Source: CAD feature listing. Evaluate the final solid. Frame: model axes, mm. Face numbers are marked on the shaded views. A direction names the side the tool comes from. Round coordinates to 2 decimals unless told otherwise and drop trailing zeros. Write each loop counter-clockwise with the first axis right and the second up, starting at its lowest first coordinate (ties: lowest second). Pieces come first, ordered by that corner, then holes. Notation, with made-up numbers: M -2.75,-22.5 L 19.25,-22.5 A34 ccw 19.25,12.5 Z; hole C 13,56 d4. An arc over 180 degrees is marked long. Answer in a Markdown table with one row per item.
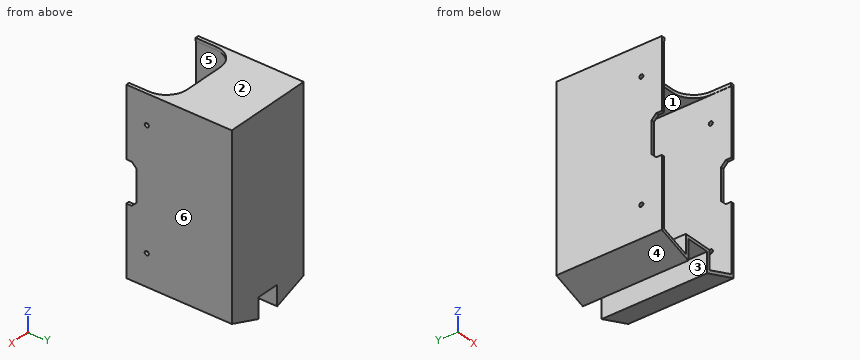
from build123d import *

# Parameters (mm, degrees)
BOSS_EXTRUDE1_DEPTH = 50
BOSS_EXTRUDE2_DEPTH = 1.52
CUT_EXTRUDE2_DEPTH  = 1.52
SKETCH4_R           = 1
CUT_EXTRUDE8_DEPTH  = 178.52
CUT_EXTRUDE9_DEPTH  = 178.52


with BuildPart() as part:
    # Sketch1 → Boss-Extrude1 (new body)
    with BuildSketch(Plane(origin=(0, 0, 0), x_dir=(1, 0, 0), z_dir=(0, 1, 0))):
        Polygon((-22.935245878, -45.076760645), (20.864754122, -45.076760645), (20.864754122, 42.660744493), (4.698193973, 48.553690828), (4.698193973, 38.723239355), (-6.768685729, 38.723239355), (-6.768685729, 48.553690828), (-22.935245878, 42.660744493), align=None)
        Polygon((-21.435245878, -43.576760645), (19.364754122, -43.576760645), (19.364754122, 41.610970221), (6.198193973, 46.410372917), (6.198193973, 37.223239355), (-8.268685729, 37.223239355), (-8.268685729, 46.410372917), (-21.435245878, 41.610970221), align=None, mode=Mode.SUBTRACT)
    extrude(amount=BOSS_EXTRUDE1_DEPTH)

    # Sketch2 → Boss-Extrude2 (add)
    with BuildSketch(Plane(origin=(0, 50, 0), x_dir=(1, 0, 0), z_dir=(0, 1, 0))):
        Polygon((-22.935245878, 42.660744493), (-22.935245878, -45.076760645), (20.864754122, -45.076760645), (20.864754122, 42.660744493), (4.698193973, 48.553690828), (4.698193973, 38.723239355), (-6.768685729, 38.723239355), (-6.768685729, 48.553690828), align=None)
    extrude(amount=BOSS_EXTRUDE2_DEPTH)

    # Sketch3 → Cut-Extrude2 (cut)
    with BuildSketch(Plane.XY.offset(45.076760645)):
        with BuildLine():
            Line((8.964754122, 20.3), (-11.035245878, 20.3))
            ThreePointArc((-11.035245878, 20.3), (-18.318445724, 17.283199846), (-21.335245878, 10))
            Line((-21.335245878, 10), (-21.335245878, -0.3))
            Line((-21.335245878, -0.3), (19.264754122, -0.3))
            Line((19.264754122, -0.3), (19.264754122, 10))
            ThreePointArc((19.264754122, 10), (16.247953968, 17.283199846), (8.964754122, 20.3))
        make_face()
    extrude(amount=-CUT_EXTRUDE2_DEPTH, mode=Mode.SUBTRACT)

    # Sketch4 → Cut-Extrude8 (cut)
    with BuildSketch(Plane(origin=(20.864754122, 0, 0), x_dir=(0, 0, -1), z_dir=(1, 0, 0))):
        with Locations((-30.703568725, 10)):
            Circle(SKETCH4_R)
        with Locations((27.32955957, 10)):
            Circle(SKETCH4_R)
    extrude(amount=-CUT_EXTRUDE8_DEPTH, mode=Mode.SUBTRACT)

    # Sketch5 → Cut-Extrude9 (cut)
    with BuildSketch(Plane(origin=(20.864754122, 0, 0), x_dir=(0, 0, -1), z_dir=(1, 0, 0))):
        Polygon((-11.208008076, 2.683848394), (-11.208008076, 0), (8.791991924, 0), (8.791991924, 2.683848394), (6.475840318, 5), (-8.89185647, 5), align=None)
    extrude(amount=-CUT_EXTRUDE9_DEPTH, mode=Mode.SUBTRACT)


solid = part.part
Q1. Pull-direction query (Z, two-part tool) for the marked faces 4, 5 and 6; classes: pulls with the +Z half, pulls with the -Z half, needs draft (parallel to the pull), parting line crosses it, or undercut.
Solutions:
| item | result |
|---|---|
| face 4 | pulls with the -Z half |
| face 5 | undercut |
| face 6 | needs draft |
Q2. Section C-C (x = 17). Return loops of the section in (y, z), and give its area (3 significant figures).
Solutions:
| item | result |
|---|---|
| outline | M 0,-44.07 L 51.52,-44.07 L 51.52,45.08 L 16.44,45.08 L 16.44,43.58 L 50,43.58 L 50,-42.47 L 0,-42.47 Z |
| area | 266 mm2 |
Q3. Contact query for flat-ended pins moving along their axis: pin 1 Ø1.5 at (x, y) = (-5, 14) entering from -Z; pin 2 Ø1.2 at (x, y) = (-22, 1) entering from -Z; pin 3 Ø2 at (x, z) = (-9.5, -33.5) entering from -Y. Output: stop coordinate, or through.
Solutions:
| item | result |
|---|---|
| pin 1 | stops at z = -38.72 |
| pin 2 | stops at z = -43.22 |
| pin 3 | stops at y = 50 |
Q4. Material intervals for probe 1 along X at (y, z) = (49.5, -40); probe 2 along X at (y, z) = (47, 23); probe 3 along Z at (x, y) = (-1, 41), sorted ascending.
Solutions:
| item | result |
|---|---|
| probe 1 | x = -22.94 to -21.44, -8.27 to -6.77, 4.7 to 6.2, 19.36 to 20.86 |
| probe 2 | x = -22.94 to -21.44, 19.36 to 20.86 |
| probe 3 | z = -38.72 to -37.22, 43.58 to 45.08 |
Q5. Section A-A (y = 36.5). Return loops of the section in (x, z).
Solutions:
| item | result |
|---|---|
| outline | M -22.94,-42.66 L -6.77,-48.55 L -6.77,-38.72 L 4.7,-38.72 L 4.7,-48.55 L 20.86,-42.66 L 20.86,45.08 L -22.94,45.08 Z; hole M -21.44,-41.61 L -8.27,-46.41 L -8.27,-37.22 L 6.2,-37.22 L 6.2,-46.41 L 19.36,-41.61 L 19.36,43.58 L -21.44,43.58 Z |
Q6. Access query for the marked faces 1, 2 and 3. Directions: +Z, -Z, +X, -X, +Y, -Y. A direction counts if a zero-diameter tool reaches every point of the face in a straight line with its end or side. Return the directions, or none.
Solutions:
| item | result |
|---|---|
| face 1 | -Y |
| face 2 | +Z, +X, -X, +Y, -Y |
| face 3 | -Z, +Y, -Y |
Q7. Section B-B (z = 0.5). Return loops of the section in (x, y), and give its area (3 significant figures).
Solutions:
| item | result |
|---|---|
| outline | M -22.94,5 L -21.44,5 L -21.44,50 L 19.36,50 L 19.36,5 L 20.86,5 L 20.86,51.52 L -22.94,51.52 Z |
| area | 202 mm2 |
